from build123d import *

# Parameters (mm, degrees)
PAD_DEPTH = 20


with BuildPart() as part:
    # Sketch → Pad (new body)
    with BuildSketch(Plane.XY):
        with BuildLine():
            Line((0, 5.5), (2, 5.5))
            ThreePointArc((2, 5.5), (3.931852, 6.982362), (3, 9.232051))
            ThreePointArc((2, 10.964102), (2.267949, 9.964102), (3, 9.232051))
            Line((2, 10.964102), (2, 20.5))
            ThreePointArc((7.5, 20.5), (4.75, 23.25), (2, 20.5))
            Line((7.5, 20.5), (7.5, 13))
            ThreePointArc((7.5, 13), (9.696699, 7.696699), (15, 5.5))
            ThreePointArc((15, 0), (17.75, 2.75), (15, 5.5))
            Line((15, 0), (0, 0))
            Line((0, 5.5), (0, 0))
        make_face()
    pad = extrude(amount=PAD_DEPTH)

    # Mirrored: Pad across Sketch V_Axis
    add(pad.mirror(Plane(origin=(0, 0, 0), x_dir=(0, 0, 1), z_dir=(1, 0, 0))))


solid = part.part
For this review, take the finished solid that the model builds, in its own axes (mm). A direction names the side the tool comes from. Round coordinates to 2 decimals unless told otherwise and drop trailing zeros. Write each loop counter-clockwise with the first axis right and the second up, starting at its lowest first coordinate (ties: lowest second). Pieces come first, ordered by that corner, then holes. Notation, with made-up numbers: (-4.5, 48) -> (3.5, 48) arc R11 cw to (3.5, 56) -> close; hole circle Ø1 at (-16.5, 58). An arc over 180 degrees is marked (long way). Use CSV: the item, a comma, the result in double quotes.
(1) Clearance check with flat-ended pins moving along their axes: P1, Ø1.2, axis at x = -1, z = 7, coming from the +Y side; P2, Ø7.5, axis at y = 16, z = 8, coming from the +X side; P3, Ø8, axis at y = 16, z = 4.5, coming from the +X side. State where each tip first meets the part, or that it passes through.
Computed values:
P1,"y = 5.5"
P2,"x = 7.54"
P3,"x = 7.57"
(2) Consider section A-A, the plane y = 14.25. Give the boundary of the cut face in (x, z).
Computed values:
outline,"(-7.5, 0) -> (-2, 0) -> (-2, 20) -> (-7.5, 20) -> close; (2, 0) -> (7.5, 0) -> (7.5, 20) -> (2, 20) -> close"
(3) To check wall thickness, follow L1, parallel to X at y = 20, z = 15; L2, parallel to X at y = 7.75, z = 6.5; L3, parallel to Y at x = -0.5, z = 14.5. State the ranges of each line that lie inside material, in increasing order. Write a range as [from, to].
Computed values:
L1,"[-7.5, -2], [2, 7.5]"
L2,"[-9.64, -3.98], [3.98, 9.64]"
L3,"[0, 5.5]"
(4) Consider section C-C, the plane x = 1. Give the boundary of the cut face in (y, z), plus the area to 3 significant figures.
Computed values:
outline,"(0, 0) -> (5.5, 0) -> (5.5, 20) -> (0, 20) -> close"
area,"110 mm²"
(5) Draft analysis for pull direction X (two halves, no side actions). For faces 4 (the face through (0, 0, 10)), 5 (the face through (-7.5, 17, 10)), 6 (the face through (-2, 16, 10)), state which applies: +X half, -X half, draft (parallel to the pull), parting line (faces both ways), or undercut.
Computed values:
face 4,"draft"
face 5,"-X half"
face 6,"undercut"
(6) Consider section B-B, the plane z = 8.5. Give the boundary of the cut face in (x, y), plus the area to 3 significant figures.
Computed values:
outline,"(-15, 0) -> (15, 0) arc R2.75 ccw to (15, 5.5) arc R7.5 cw to (7.5, 13) -> (7.5, 20.5) arc R2.75 ccw to (2, 20.5) -> (2, 10.96) arc R2 ccw to (3, 9.23) arc R2 cw to (2, 5.5) -> (-2, 5.5) arc R2 cw to (-3, 9.23) arc R2 ccw to (-2, 10.96) -> (-2, 20.5) arc R2.75 ccw to (-7.5, 20.5) -> (-7.5, 13) arc R7.5 cw to (-15, 5.5) arc R2.75 ccw to start"
area,"388 mm²"
(7) Consider section D-D, the plane y = 10.5. Give the boundary of the cut face in (x, z), plus the area to 3 significant figures.
Computed values:
outline,"(-7.93, 0) -> (-2.05, 0) -> (-2.05, 20) -> (-7.93, 20) -> close; (2.05, 0) -> (7.93, 0) -> (7.93, 20) -> (2.05, 20) -> close"
area,"235 mm²"
(8) For faces 1 (the face through (2, 16, 10)), 2 (the face through (7.5, 17, 10)), 3 (the face through (17.75, 2.69, 9.86)), list the 3-axis set-ups (+Z, -Z, +X, -X, +Y, -Y) from which the entire face can be reached by the end or side of a thin tool; tool diameter is ignored.
Computed values:
face 1,"+Z, -Z, +Y"
face 2,"+Z, -Z, +X, +Y"
face 3,"+Z, -Z, +X"
